Read the model definition and answer for the solid it produces. Units are mm, in the model's axes. A direction names the side the tool comes from. Coordinates: 2 decimals unless noted, no trailing zeros. Loops run counter-clockwise (first coordinate to the right, second up) from the corner with the lowest first, then second, coordinate; pieces in that order, holes last. Notation, with made-up numbers: (3, 63) -> (25, 63) arc R22 cw to (25, 100) -> close; hole circle Ø1 at (35.5, -39.5). An arc over 180 degrees is marked (long way). Answer as a JSON object with one key per item and string values. Group by question number.
Q1. Determine the mould class of faces 1 (the cylindrical face through (-154.58, -219.05, -8.67)), 2 (the flat face through (-185, -146, -22)), 3 (the flat face through (-1, -179, 125)) for opening direction X: released by +X, released by -X, zero draft, split by the parting line, or undercut.
Q2. Straight lines are drawn through the part: line 1 along Y through (x, z) = (-151, 0); line 2 along Z through (x, y) = (184.5, -246); line 3 along Y through (x, z) = (143.5, -15.5). For each, find the intervals that lie inside material, in ascending order. Write a range as [from, to].
Q3. The part is cut by section C-C on y = -330. Write down the section's boundary in (x, z).
Q4. Each of these flat-tipped pins is pushed along its axis until it touches: P1, Ø3, axis at y = -214.5, z = -112.5, coming from the +X side; P2, Ø5, axis at y = -302.5, z = 65.5, coming from the -X side; P3, Ø12, axis at y = -245.5, z = 89.5, coming from the +X side. Where does it stop, or does it pass through?
Q5. The part is cut by section B-B on y = -70.5. Write down the section's boundary in (x, z).
Q6. For faces 4 (the cylindrical face through (154.58, -262.979, 18.426)), 5 (the flat face through (99, -202, 125)), 6 (the flat face through (-22, -146, 185)), 7 (the flat face through (22, -146, -185)), determine the directions among +Z, -Z, +X, -X, +Y, -Y from which every point of the face is accessible in a straight line to the end or side of a thin tool.
Q7. The part is cut by section A-A on x = 158. Write down the section's boundary in (y, z), and give its area (3 significant figures).
from build123d import *

# Parameters (mm, degrees)
SKETCH1_R           = 100
BOSS_EXTRUDE1_DEPTH = 80
SKETCH2_W           = 250
SKETCH2_H           = 250
BOSS_EXTRUDE2_DEPTH = 200
SKETCH3_R           = 80
SKETCH3_R_2         = 70
BOSS_EXTRUDE3_DEPTH = 100
CHAMFER1_SIZE       = 20
SKETCH4_W           = 20
SKETCH4_H           = 200
CUT_EXTRUDE1_DEPTH  = 20
SKETCH5_R           = 100
SKETCH5_R_2         = 90
BOSS_EXTRUDE4_DEPTH = 80
SKETCH6_R           = 85
SKETCH6_R_2         = 75
SKETCH6_R_3         = 50
SKETCH6_R_4         = 40
BOSS_EXTRUDE5_DEPTH = 60
CIRPATTERN1_COUNT   = 4
FILLET1_R           = 10
SKETCH7_R           = 12.5
CUT_EXTRUDE2_DEPTH  = 123


with BuildPart() as part:
    # Sketch1 → Boss-Extrude1 (new body)
    with BuildSketch(Plane(origin=(0, 0, 0), x_dir=(1, 0, 0), z_dir=(0, 1, 0))):
        Circle(SKETCH1_R)
    extrude(amount=-BOSS_EXTRUDE1_DEPTH)

    # Sketch2 → Boss-Extrude2 (add)
    with BuildSketch(Plane.XZ.offset(80)):
        Rectangle(SKETCH2_W, SKETCH2_H)
    extrude(amount=BOSS_EXTRUDE2_DEPTH)

    # Sketch3 → Boss-Extrude3 (add)
    with BuildSketch(Plane.XZ.offset(280)):
        Circle(SKETCH3_R)
        Circle(SKETCH3_R_2, mode=Mode.SUBTRACT)
    extrude(amount=BOSS_EXTRUDE3_DEPTH)

    # Chamfer1
    chamfer1_edges = [part.edges().sort_by_distance(p)[0] for p in [
        (-100, 0, 0),
        (-100, -80, 0),
    ]]
    chamfer(chamfer1_edges, length=CHAMFER1_SIZE)

    # Sketch4 → Cut-Extrude1 (cut)
    with BuildSketch(Plane(origin=(125, 0, 0), x_dir=(0, 0, -1), z_dir=(1, 0, 0))):
        with Locations((-115, -180)):
            Rectangle(SKETCH4_W, SKETCH4_H)
        with Locations((115, -180)):
            Rectangle(SKETCH4_W, SKETCH4_H)
    cut_extrude1 = extrude(amount=-CUT_EXTRUDE1_DEPTH, mode=Mode.SUBTRACT)

    # Sketch5 → Boss-Extrude4 (add)
    with BuildSketch(Plane(origin=(125, 0, 0), x_dir=(0, 0, -1), z_dir=(1, 0, 0))):
        with Locations((0, -180)):
            Circle(SKETCH5_R)
        with Locations((0, -180)):
            Circle(SKETCH5_R_2, mode=Mode.SUBTRACT)
    boss_extrude4 = extrude(amount=BOSS_EXTRUDE4_DEPTH)

    # Sketch6 → Boss-Extrude5 (add)
    with BuildSketch(Plane(origin=(125, 0, 0), x_dir=(0, 0, -1), z_dir=(1, 0, 0))):
        with Locations((0, -180)):
            Circle(SKETCH6_R)
        with Locations((0, -180)):
            Circle(SKETCH6_R_2, mode=Mode.SUBTRACT)
        with Locations((0, -180)):
            Circle(SKETCH6_R_3)
        with Locations((0, -180)):
            Circle(SKETCH6_R_4, mode=Mode.SUBTRACT)
    boss_extrude5 = extrude(amount=BOSS_EXTRUDE5_DEPTH)

    # CirPattern1: Cut-Extrude1, Boss-Extrude4, Boss-Extrude5 ×4 about axis
    cirpattern1_axis = Axis((0, 0, 0), (0, 1, 0))
    for i in range(1, CIRPATTERN1_COUNT):
        add(cut_extrude1.rotate(cirpattern1_axis, i * 360 / CIRPATTERN1_COUNT), mode=Mode.SUBTRACT)
        add(boss_extrude4.rotate(cirpattern1_axis, i * 360 / CIRPATTERN1_COUNT))
        add(boss_extrude5.rotate(cirpattern1_axis, i * 360 / CIRPATTERN1_COUNT))

    # Fillet1
    fillet1_edges = [part.edges().sort_by_distance(p)[0] for p in [
        (-105, -180, 105),
        (-105, -180, -105),
        (105, -180, 105),
        (105, -180, -105),
    ]]
    fillet(fillet1_edges, radius=FILLET1_R)

    # Sketch7 → Cut-Extrude2 (cut)
    with BuildSketch(Plane.XY):
        with Locations((0, -330)):
            Circle(SKETCH7_R)
    extrude(amount=-CUT_EXTRUDE2_DEPTH, mode=Mode.SUBTRACT)


solid = part.part
Final values:
{
 "1": {"face 1": "zero draft", "face 2": "released by -X", "face 3": "undercut"},
 "2": {"line 1": "y = [-280, -270], [-265, -255], [-230, -220], [-140, -130], [-105, -95], [-90, -80]", "line 2": "z = [-75.13, -61.19], [-53.56, -35.62], [35.62, 53.56], [61.19, 75.13]", "line 3": "y = [-278.79, -268.66], [-263.57, -253.38], [-227.54, -216.87], [-143.13, -132.46], [-106.62, -96.43], [-91.34, -81.21]"},
 "3": {"outline": "(-12.5, -79.02) -> (-12.5, -68.87) arc R70 cw (long way) to (12.5, -68.87) -> (12.5, -79.02) arc R80 ccw (long way) to start"},
 "4": {"P1": "stops at x = 105.83", "P2": "stops at x = -49.31", "P3": "stops at x = 125"},
 "5": {"outline": "circle Ø221 at (0, 0)"},
 "6": {"face 4": "+X", "face 5": "+Z, +X", "face 6": "+Z", "face 7": "-Z"},
 "7": {"outline": "circle Ø200 at (-180, 0); circle Ø170 at (-180, 0); circle Ø100 at (-180, 0); hole circle Ø180 at (-180, 0); hole circle Ø150 at (-180, 0); hole circle Ø80 at (-180, 0)", "area": "13,800 mm2"}
}
